```python
from build123d import *

# Parameters (mm, degrees)
F0_W        = 30
F0_H        = 10
F0_W_2      = 10.3326633751
F1_DEPTH    = 600
F2_T1_DEPTH = 1362.4185197182
F3_SIZE2    = 149.99999
F3_SIZE     = 24.99999
F4_R        = 2.5


# Not quite as in the source:
# - a fillet or chamfer that OpenCascade refuses, or shapes differently, is made with other operations: its cross-section is extruded or revolved along the edge and cut away or added
# - a fillet or chamfer is up to 0.001 mm smaller than in the source, because OpenCascade refuses the exact size


with BuildPart() as f1:
    # F0 (on Front) → F1 (new body)
    with BuildSketch(Plane.XZ):
        Polygon((0, -10), (0, 0), (-150, 0), (-150, -30), (0, -30), (0, -20), align=None)
        with Locations((75.3326633751, -15)):
            Rectangle(F0_W, F0_H)
        with Locations((5.1663316875, -15)):
            Rectangle(F0_W_2, F0_H)
        with Locations((35.3326633751, -15)):
            Rectangle(F0_W, F0_H)
        Polygon((10.3326633751, -20), (0, -20), (0, -30), (100.4177228767, -30), (100.4177228767, -20), (90.3326633751, -20), (60.3326633751, -20), (50.3326633751, -20), (20.3326633751, -20), align=None)
        Polygon((100.4177228767, -20), (100.4177228767, -30), (110.4177228767, -30), (110.4177228767, -10), (100.4177228767, -10), align=None)
    extrude(amount=F1_DEPTH)

    # F2: chamfer of 261 on 1 edges, made by hand

    # F2_s2 → F2_t1 (cut)
    with BuildSketch(Plane.XY.offset(-701.2092598591)):
        Polygon((110.4177228767, -339), (-150.5822771233, -600), (110.4177228767, -600), align=None)
    extrude(amount=F2_T1_DEPTH, mode=Mode.SUBTRACT)

    # F3 (size 25 and 150 in the source; OpenCascade refuses exactly that, so slightly less here)
    f3_edges = [f1.edges().sort_by_distance(p)[0] for p in [
        (-150, -299.708861, 0),
    ]]
    f3_side = f1.faces().sort_by_distance((-150, -299.708861, -15))[0]
    chamfer(f3_edges, length=F3_SIZE, length2=F3_SIZE2, reference=f3_side)

    # F4
    f4_edges = [f1.edges().sort_by_distance(p)[0] for p in [
        (-150, -299.708861, -24.99999),
        (-150, -299.708861, -30),
    ]]
    fillet(f4_edges, radius=F4_R)

    # F5: F1 across face


with BuildPart() as f1_1:
    add(f1.part)
    add(f1.part.mirror(Plane(origin=(-9.807206416, -459.2249292927, -20.1902158269), x_dir=(0.7071067812, 0.7071067812, 0), z_dir=(0.7071067812, -0.7071067812, 0))))


solid = f1_1.part
```
Work out the finished part from the listing and answer in its coordinate system (mm). A direction names the side the tool comes from. Round coordinates to 2 decimals unless told otherwise and drop trailing zeros. Loops run counter-clockwise (first coordinate to the right, second up) from the corner with the lowest first, then second, coordinate; pieces in that order, holes last. Notation, with made-up numbers: M -6,9 L 11,9 A32 ccw 11,41 Z; hole C 5.5,-4 d1. An arc over 180 degrees is marked long. Use CSV: the item, a comma, the result in double quotes.
Q1. The mould has two halves that part along X. Classify faces 1 (the flat face through (126, -442, -10)), 2 (the flat face through (-72.92, -228.113, -12.153)), 3 (the flat face through (191, -352, -20)): pulls with the +X half, pulls with the -X half, needs draft (parallel to the pull), parting line crosses it, or undercut.
Determined:
face 1,"needs draft"
face 2,"pulls with the -X half"
face 3,"undercut"
Q2. Each of these flat-tipped pins is pushed along its axis until it touches: pin 1 (5 mm diameter, centred on y = -158.5, z = -17.5, fed in from +X); pin 2 (8 mm diameter, centred on x = 81, z = -3, fed in from +Y); pin 3 (3 mm diameter, centred on y = -257, z = -7.5, fed in from +X). Where does it stop, or does it pass through?
Determined:
pin 1,"x = 110.42"
pin 2,"y = -449.42"
pin 3,"x = 0"
Q3. Section C-C, the plane y = -550.5 is taken. Determine the outline of the cut face in (x, z).
Determined:
outline,"M -150,-27.5 A2.5 ccw -147.5,-30 L 449.42,-30 L 449.42,-16.85 L -101.08,-16.85 L -147.91,-24.65 A2.5 ccw -150,-27.12 Z"
Q4. A tool of negligible diameter and unlimited length cuts with its end or side. For faces 4 (the flat face through (221.305, -522.338, -12.153)), 5 (the flat face through (198, -342, -10)), 6 (the flat face through (282, -339, -20)), from which of +Z, -Z, +X, -X, +Y, -Y can it reach the whole face along a straight path? Write none if from no direction.
Determined:
face 4,"+Z, +X, -X, -Y"
face 5,"+Z, +X, +Y"
face 6,"+Z, -Z, +X, +Y"
Q5. Consider L1, parallel to Y at x = 409.5, z = -27; L2, parallel to Z at x = 357.5, y = -383; L3, parallel to Z at x = 15, y = -351. Determine where each line is inside the solid, lowest interval first.
Determined:
L1,"-599.41 to -339"
L2,"-30 to -10"
L3,"-30 to -20"
